The drawing under review shows one solid part. Ordinate dimensions are in mm from its lowest x, y, z. Give positions to 0.01 mm unless a question says otherwise; leave off trailing zeros. Write each loop counter-clockwise with the first axis right and the second up, starting at its lowest first coordinate (ties: lowest second). Pieces come first, ordered by that corner, then holes. Notation, with made-up numbers: M 23.25,58 L 43.25,58 A37 cw 43.25,96 Z; hole C -33,-6.5 d6. An arc over 180 degrees is marked long. One line per item, written item: value. Start each with the question number.
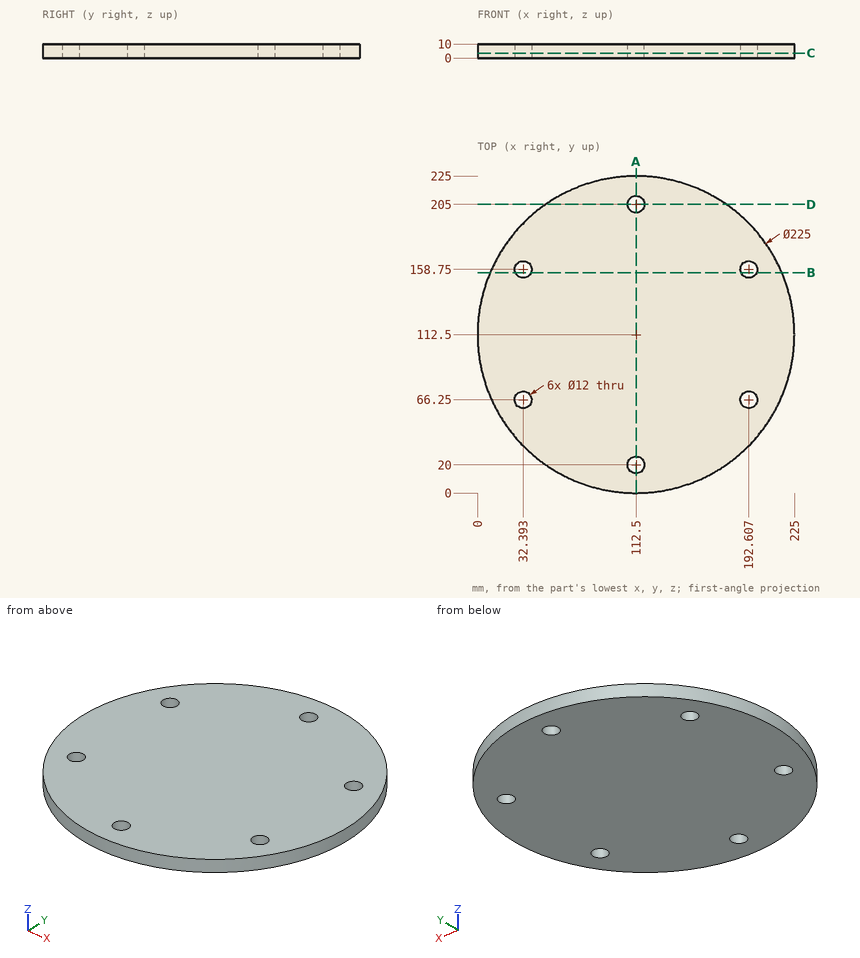
Q1. Take a section at A-A, the plane x = 112.5. Give the boundary of the cut face in (y, z), then the cut area to 3 significant figures.
Q2. Take a section at B-B, the plane y = 156.5. Give the boundary of the cut face in (x, z) (1 decimal).
Q3. Take a section at D-D, the plane y = 205. Give the boundary of the cut face in (x, z).
Q4. Wall thickness on line 1 (Y direction, x = 112.5, z = 4.75); line 2 (Y direction, x = 28.5, z = 5.75) (1 decimal); line 3 (X direction, y = 64, z = 5.5) (1 decimal): over which ranges is each line inside the solid? List them lowest first. Write a range as from..to.
Q5. Take a section at C-C, the plane z = 3.5. Give the boundary of the cut face in (x, y).
Q6. For P1, Ø7, axis at x = 32.39, y = 66.25, coming from the -Z side; P2, Ø2, axis at y = 70, z = 6, coming from the +X side (1 decimal); P3, Ø1.5, axis at y = 39.5, z = 8, coming from the -X side; P4, Ø1, axis at y = 119.5, z = 2.5, coming from the -X side, all flat-tipped, find the tip position at first contact; note any pin that passes through.
Results list:
1. outline: M 0,0 L 14,0 L 14,10 L 0,10 Z; M 26,0 L 199,0 L 199,10 L 26,10 Z; M 211,0 L 225,0 L 225,10 L 211,10 Z
1. area: 2,010 mm^2
2. outline: M 9,0 L 26.8,0 L 26.8,10 L 9,10 Z; M 38,0 L 187,0 L 187,10 L 38,10 Z; M 198.2,0 L 216,0 L 216,10 L 198.2,10 Z
3. outline: M 48.47,0 L 106.5,0 L 106.5,10 L 48.47,10 Z; M 118.5,0 L 176.53,0 L 176.53,10 L 118.5,10 Z
4. line 1: y = 0..14, 26..199, 211..225
4. line 2: y = 37.7..61.7, 70.8..154.2, 163.3..187.3
4. line 3: x = 11..26.8, 38..187, 198.2..214
5. outline: C 112.5,112.5 d225; hole C 32.39,66.25 d12; hole C 32.39,158.75 d12; hole C 112.5,20 d12; hole C 112.5,205 d12; hole C 192.61,66.25 d12; hole C 192.61,158.75 d12
6. P1: passes through
6. P2: stops at x = 217.1
6. P3: stops at x = 26.27
6. P4: stops at x = 0.19
